from build123d import *

# Parameters (mm, degrees)
SKETCH1_W           = 113
SKETCH1_H           = 55
BOSS_EXTRUDE1_DEPTH = 6
BOSS_EXTRUDE3_DEPTH = 113
SKETCH2_R           = 2.25
BOSS_EXTRUDE2_DEPTH = 5
SHELL1_START        = -50.038745387
SHELL1_DEPTH        = 108
SKETCH4_W           = 44
SKETCH4_H           = 7
SKETCH4_W_2         = 88
SKETCH4_H_2         = 40.5
CUT_EXTRUDE1_DEPTH  = 10
FILLET2_R           = 3.5
CUT_EXTRUDE2_START  = -52.5
SKETCH5_W           = 45
SKETCH5_H           = 7
CUT_EXTRUDE2_DEPTH  = 52.5
FILLET3_R           = 3


# Read off the part's stored shape, not the designer's step: Shell1
with BuildPart() as part:
    # Sketch1 → Boss-Extrude1 (new body)
    with BuildSketch(Plane(origin=(0, 0, 0), x_dir=(1, 0, 0), z_dir=(0, 1, 0))):
        with Locations((3.961254613, 12.529520295)):
            Rectangle(SKETCH1_W, SKETCH1_H)
    extrude(amount=BOSS_EXTRUDE1_DEPTH)

    # Sketch3 → Boss-Extrude3 (add)
    with BuildSketch(Plane(origin=(60.461254613, 0, 0), x_dir=(0, 0, -1), z_dir=(1, 0, 0))):
        Polygon((-14.970479705, 0), (-14.970479705, -50.990195136), (40.029520295, 0), align=None)
    extrude(amount=-BOSS_EXTRUDE3_DEPTH)

    # Sketch2 → Boss-Extrude2 (add)
    with BuildSketch(Plane(origin=(0, 6, 0), x_dir=(1, 0, 0), z_dir=(0, 1, 0))):
        with Locations(Location((-46.038745387, 31.709520295, 0), (0, 0, 270))):
            Circle(SKETCH2_R)
        with Locations(Location((53.961254613, 31.629520295, 0), (0, 0, 270))):
            Circle(SKETCH2_R)
        with Locations(Location((53.961254613, 1.029520295, 0), (0, 0, 270))):
            Circle(SKETCH2_R)
        with Locations(Location((-46.038745387, 1.029520295, 0), (0, 0, 270))):
            Circle(SKETCH2_R)
    extrude(amount=BOSS_EXTRUDE2_DEPTH)

    # Shell1 outline → Shell1 (cut)
    with BuildSketch(Plane.YZ.offset(SHELL1_START)):
        Polygon((3.5, 12.470479705), (-48.672458993, 12.470479705), (-2.317736143, -37.529520295), (3.5, -37.529520295), align=None)
    extrude(amount=SHELL1_DEPTH, mode=Mode.SUBTRACT)

    # Sketch4 → Cut-Extrude1 (cut)
    with BuildSketch(Plane.XZ.offset(-3.5)):
        with Locations((25.961254613, -34.029520295)):
            Rectangle(SKETCH4_W, SKETCH4_H)
        with Locations((3.961254613, -10.279520295)):
            Rectangle(SKETCH4_W_2, SKETCH4_H_2)
    extrude(amount=-CUT_EXTRUDE1_DEPTH, mode=Mode.SUBTRACT)

    # Fillet2
    fillet2_edges = [part.edges().sort_by_distance(p)[0] for p in [
        (-52.538745387, 3, -40.029520295),
        (60.461254613, 3, -40.029520295),
        (60.461254613, -22.495097568, 14.970479705),
        (-52.538745387, -22.495097568, 14.970479705),
    ]]
    fillet(fillet2_edges, radius=FILLET2_R)

    # Sketch5 → Cut-Extrude2 (cut)
    with BuildSketch(Plane.XY.offset(14.970479705).offset(CUT_EXTRUDE2_START)):
        with Locations((26.461254613, 2.5)):
            Rectangle(SKETCH5_W, SKETCH5_H)
    extrude(amount=CUT_EXTRUDE2_DEPTH, mode=Mode.SUBTRACT)

    # Fillet3
    fillet3_edges = [part.edges().sort_by_distance(p)[0] for p in [
        (3.961254613, -1, 13.720479705),
        (48.961254613, -1, 13.720479705),
    ]]
    fillet(fillet3_edges, radius=FILLET3_R)


solid = part.part
Build history of the part. All positions in model axes, mm. A direction names the side the tool comes from. Round coordinates to 2 decimals unless told otherwise and drop trailing zeros. Write each loop counter-clockwise with the first axis right and the second up, starting at its lowest first coordinate (ties: lowest second). Pieces come first, ordered by that corner, then holes. Notation, with made-up numbers: M 80,61.5 L 94,61.5 A9 cw 94,75.5 Z; hole C 11.25,27 d3. An arc over 180 degrees is marked long. Answer as a JSON object with one key per item and string values. Group by question number.
(1) Cut at D-D (x = 37.5). Give the cut face in (y, z).
(2) Cut at C-C (y = -12.5). Give the cut face in (x, z).
(3) Which spindle directions (+Z, -Z, +X, -X, +Y, -Y) get a long thin tool onto all of the face, cutting with end or side? Do faces 4 (the flat face through (-40.039, 5, -11)), 5 (the cylindrical face through (-48.035, 8.465, 0.009)), 6 (the flat face through (-41, 3.5, -14)), 7 (the cylindrical face through (4.86, -0.14, 13.74)). Say none if no direction does.
(4) Flat gauge pins, fed straight in: pin 1 (4 mm diameter, centred on y = -42, z = 3, fed in from -X); pin 2 (1.3 mm diameter, centred on x = 35, z = 14, fed in from +Y); pin 3 (6 mm diameter, centred on x = 11, y = -26, fed in from -Z); pin 4 (10 mm diameter, centred on x = 51.5, z = -24, fed in from -Y). Where does each tip first touch, or does it go through?
(5) Cut at B-B (z = -16.5). Give the cut face in (x, y).
(6) Cut at A-A (x = -38). Give the cut face in (y, z), and give its area (3 significant figures).
(7) Drill centre lines: L1, parallel to X at y = -24, z = -12.5; L2, parallel to Z at x = -4, y = 0; L3, parallel to Z at x = -33, y = -42. Where is each one in solid material? Low to high.
(8) Mould opens along Z. For faces 1 (the cylindrical face through (59.41, -22.1, 13.97)), 2 (the cylindrical face through (-46.9, 8.46, -29.63)), 3 (the flat face through (26, -1, 14)) say: pulls with the +Z half, pulls with the -Z half, needs draft (parallel to the pull), parting line crosses it, or undercut.
Responses:
{
 "1": {"outline": "M -50.99,14.97 L -48.67,12.47 L -1,12.47 L -1,14.97 Z; M -2.32,-37.53 L 0,-40.03 L 6,-40.03 L 6,-37.53 Z"},
 "2": {"outline": "M -52.54,-26.55 L -50.04,-26.55 L -50.04,12.47 L 57.96,12.47 L 57.96,-26.55 L 60.46,-26.55 L 60.46,11.47 A3.5 ccw 56.96,14.97 L -49.04,14.97 A3.5 ccw -52.54,11.47 Z"},
 "3": {"face 4": "+Y, -Y", "face 5": "+Y", "face 6": "-Y", "face 7": "+Z, +Y"},
 "4": {"pin 1": "stops at x = -52.54", "pin 2": "stops at y = -1", "pin 3": "stops at z = 12.47", "pin 4": "stops at y = 3.5"},
 "5": {"outline": "M -52.54,-21.81 L -50.04,-21.81 L -50.04,3.5 L -40.04,3.5 L -40.04,6 L -52.54,6 Z; M 48.96,3.5 L 57.96,3.5 L 57.96,-21.81 L 60.46,-21.81 L 60.46,6 L 48.96,6 Z"},
 "6": {"outline": "M -50.99,14.97 L -48.67,12.47 L 3.5,12.47 L 3.5,9.97 L 6,9.97 L 6,14.97 Z; M -2.32,-37.53 L 0,-40.03 L 6,-40.03 L 6,-30.53 L 3.5,-30.53 L 3.5,-37.53 Z", "area": "181 mm2"},
 "7": {"L1": "x = -52.54 to -50.04, 57.96 to 60.46", "L2": "z = -40.03 to -37.53, 12.47 to 14.97", "L3": "z = 12.47 to 14.97"},
 "8": {"face 1": "pulls with the +Z half", "face 2": "undercut", "face 3": "needs draft"}
}
